```python
from build123d import *

# Parameters (mm, degrees)
SKETCH2_R                = 48.5
BOSS_EXTRUDE1_DEPTH      = 4
SKETCH4_R                = 1.5
CUT_EXTRUDE2_DEPTH       = 5
SKETCH5_R                = 3.75
CUT_EXTRUDE3_DEPTH       = 1.5
BOSS_EXTRUDE2_DEPTH      = 14
CUT_EXTRUDE5_REACH       = 44.5
SKETCH9_R                = 1.3
CUT_EXTRUDE6_DEPTH       = 7.5
CUT_EXTRUDE9_REACH       = 46.5
SKETCH11_R               = 9
BOSS_EXTRUDE7_DEPTH      = 9
BOSS_EXTRUDE7_DEPTH_BACK = 14
BOSS_EXTRUDE10_DEPTH     = 9
SKETCH27_W               = 16
SKETCH27_H               = 6
BOSS_EXTRUDE11_DEPTH     = 12
FILLET6_R                = 3
CUT_EXTRUDE16_REACH      = 75.05
SKETCH28_W               = 8
SKETCH28_H               = 4
CUT_EXTRUDE17_DEPTH      = 49.5
CUT_EXTRUDE17_DEPTH_BACK = 49.5
CROQUIS4_W               = 5.1
CROQUIS4_H               = 22.5
SALIENTE_EXTRUIR1_DEPTH  = 45
CROQUIS5_W               = 1.7
CROQUIS5_H               = 19.2
CORTAR_EXTRUIR1_DEPTH    = 19.5
CROQUIS6_W               = 18
CROQUIS6_H               = 17.447039648
CORTAR_EXTRUIR2_DEPTH    = 19.5
REDONDEO1_R              = 3
CROQUIS7_R               = 1.99
CORTAR_EXTRUIR3_DEPTH    = 10
CROQUIS8_W               = 0.564126112
CROQUIS8_H               = 2.164439882
SALIENTE_EXTRUIR2_DEPTH  = 3


with BuildPart() as part:
    # Sketch2 → Boss-Extrude1 (new body)
    with BuildSketch(Plane(origin=(0, 0, 0), x_dir=(1, 0, 0), z_dir=(0, 1, 0))):
        Circle(SKETCH2_R)
    extrude(amount=BOSS_EXTRUDE1_DEPTH)

    # Sketch4 → Cut-Extrude2 (cut, through all)
    with BuildSketch(Plane.XZ):
        with Locations((0, 7.25)):
            Circle(SKETCH4_R)
        with Locations((0, -7.25)):
            Circle(SKETCH4_R)
    extrude(amount=-CUT_EXTRUDE2_DEPTH, mode=Mode.SUBTRACT)

    # Sketch5 → Cut-Extrude3 (cut)
    with BuildSketch(Plane.XZ):
        Circle(SKETCH5_R)
    extrude(amount=-CUT_EXTRUDE3_DEPTH, mode=Mode.SUBTRACT)

    # Sketch7 → Boss-Extrude2 (add)
    with BuildSketch(Plane(origin=(-4, 0, 0), x_dir=(0, 0, -1), z_dir=(1, 0, 0))):
        with BuildLine():
            Line((23.129947874, 4), (23.129947874, 11.644549616))
            ThreePointArc((23.129947874, 11.644549616), (24.589048403, 18.743749901), (28.729797284, 24.692011643))
            ThreePointArc((28.729797284, 24.692011643), (29.313383054, 55.284736897), (-1.284289494, 55.479275971))
            Line((-1.284289494, 55.479275971), (-27.227315747, 29.536249718))
            ThreePointArc((-27.227315747, 29.536249718), (-32.64663453, 21.425665997), (-34.549646217, 11.858580188))
            Line((-34.549646217, 11.858580188), (-34.549646217, 4))
            Line((-34.549646217, 4), (23.129947874, 4))
        make_face()
    extrude(amount=-BOSS_EXTRUDE2_DEPTH)

    # Sketch8 → Cut-Extrude5 (cut, up to next)
    with BuildSketch(Plane(origin=(-6, 0, 0), x_dir=(0, 0, -1), z_dir=(1, 0, 0)), mode=Mode.PRIVATE) as cut_extrude5_sk1:
        Polygon((-15.249648422, 25.957567857), (13.741729607, 54.948945886), (28.590972012, 40.099703481), (-0.400406017, 11.108325452), align=None)
    cut_extrude5_tool1 = extrude(cut_extrude5_sk1.sketch, amount=-CUT_EXTRUDE5_REACH, mode=Mode.PRIVATE) & part.part
    add(cut_extrude5_tool1.solids().sort_by_distance((-6, 33.028636, -6.670662))[0], mode=Mode.SUBTRACT)

    # Sketch9 → Cut-Extrude6 (cut)
    with BuildSketch(Plane.ZY.offset(18)):
        with Locations((-20.105690637, 53.534732323)):
            Circle(SKETCH9_R)
        with Locations((-27.176758449, 46.463664511)):
            Circle(SKETCH9_R)
        with Locations((6.764367048, 12.522539014)):
            Circle(SKETCH9_R)
        with Locations((13.83543486, 19.593606826)):
            Circle(SKETCH9_R)
    extrude(amount=-CUT_EXTRUDE6_DEPTH, mode=Mode.SUBTRACT)

    # Sketch11 → Cut-Extrude9 (cut, up to next)
    with BuildSketch(Plane(origin=(-4, 0, 0), x_dir=(0, 0, -1), z_dir=(1, 0, 0)), mode=Mode.PRIVATE) as cut_extrude9_sk1:
        with Locations((13.918506302, 40.276480176)):
            Circle(SKETCH11_R)
    cut_extrude9_tool1 = extrude(cut_extrude9_sk1.sketch, amount=-CUT_EXTRUDE9_REACH, mode=Mode.PRIVATE) & part.part
    add(cut_extrude9_tool1.solids().sort_by_distance((-4, 40.27648, -13.918506))[0], mode=Mode.SUBTRACT)

    # Sketch17 → Boss-Extrude7 (add, two sides)
    with BuildSketch(Plane.ZY.offset(18)) as boss_extrude7_sk:
        with BuildLine():
            ThreePointArc((34.549646217, 11.858580188), (33.008342843, 20.500891953), (28.574482006, 28.077569775))
            ThreePointArc((28.574482006, 28.077569775), (27.915386359, 28.820289685), (27.227315747, 29.536249718))
            Line((27.227315747, 29.536249718), (1.284289494, 55.479275971))
            Line((1.284289494, 55.479275971), (26.295003593, 26.127182305))
            ThreePointArc((26.295003593, 26.127182305), (30.194232218, 19.461281607), (31.549646217, 11.858580188))
            Line((31.549646217, 11.858580188), (31.549646217, 4))
            Line((31.549646217, 4), (34.549646217, 4))
            Line((34.549646217, 4), (34.549646217, 11.858580188))
        make_face()
        with BuildLine():
            Line((28.574482006, 28.077569775), (3.405609837, 57.600596315))
            ThreePointArc((3.405609837, 57.600596315), (-31.461505391, 57.378912253), (-30.796489049, 22.517434639))
            ThreePointArc((-30.796489049, 22.517434639), (-27.345864981, 17.560549854), (-26.129947874, 11.644549616))
            Line((-26.129947874, 11.644549616), (-26.129947874, 4))
            Line((-26.129947874, 4), (-23.129947874, 4))
            Line((-23.129947874, 4), (-23.129947874, 11.644549616))
            ThreePointArc((-23.129947874, 11.644549616), (-24.589048403, 18.743749901), (-28.729797284, 24.692011643))
            ThreePointArc((-28.729797284, 24.692011643), (-29.313383054, 55.284736897), (1.284289494, 55.479275971))
            Line((1.284289494, 55.479275971), (27.227315747, 29.536249718))
            ThreePointArc((27.227315747, 29.536249718), (27.915386359, 28.820289685), (28.574482006, 28.077569775))
        make_face()
    extrude(amount=BOSS_EXTRUDE7_DEPTH)
    extrude(boss_extrude7_sk.sketch, amount=-BOSS_EXTRUDE7_DEPTH_BACK)

    # Sketch25 → Boss-Extrude10 (add)
    with BuildSketch(Plane.ZY.offset(18)):
        with BuildLine():
            ThreePointArc((-28.729797284, 24.692011643), (-24.589048403, 18.743749901), (-23.129947874, 11.644549616))
            Line((-23.129947874, 11.644549616), (-23.129947874, 4))
            Line((-23.129947874, 4), (-15.129947874, 4))
            add(Edge.make_bspline(
                [(-28.729797284, 24.692011643), (-21.954867515, 18.253200081), (-19.09405247, 12.798017691), (-15.129947874, 4)],
                knots=[0, 0, 0, 0, 1, 1, 1, 1], degree=3))
        make_face()
        with BuildLine():
            add(Edge.make_bspline(
                [(11.751619577, 43.19501844), (26.551255916, 25.8264495), (25.549646217, 4)],
                knots=[0, 0, 0, 1, 1, 1], degree=2))
            Line((25.549646217, 4), (31.549646217, 4))
            Line((31.549646217, 4), (31.549646217, 11.858580188))
            ThreePointArc((31.549646217, 11.858580188), (30.194232218, 19.461281607), (26.295003593, 26.127182305))
            Line((26.295003593, 26.127182305), (11.751619577, 43.19501844))
        make_face()
    extrude(amount=BOSS_EXTRUDE10_DEPTH)

    # Sketch27 → Boss-Extrude11 (add)
    with BuildSketch(Plane(origin=(0, 4, 0), x_dir=(1, 0, 0), z_dir=(0, 1, 0))):
        with Locations((6, -21.549646217)):
            Rectangle(SKETCH27_W, SKETCH27_H)
    extrude(amount=BOSS_EXTRUDE11_DEPTH)

    # Fillet6
    fillet6_edges = [part.edges().sort_by_distance(p)[0] for p in [
        (-2, 16, 21.549646217),
        (14, 16, 21.549646217),
    ]]
    fillet(fillet6_edges, radius=FILLET6_R)

    # Sketch28 → Cut-Extrude16 (cut, up to next)
    with BuildSketch(Plane.XY.offset(24.549646217), mode=Mode.PRIVATE) as cut_extrude16_sk1:
        with Locations((6, 10)):
            Rectangle(SKETCH28_W, SKETCH28_H)
    cut_extrude16_tool1 = extrude(cut_extrude16_sk1.sketch, amount=-CUT_EXTRUDE16_REACH, mode=Mode.PRIVATE) & part.part
    add(cut_extrude16_tool1.solids().sort_by_distance((6, 10, 24.549646))[0], mode=Mode.SUBTRACT)

    # Sketch29 → Cut-Extrude17 (cut, two sides)
    with BuildSketch(Plane.XY) as cut_extrude17_sk:
        with BuildLine():
            Line((-21, 64.776480176), (-27, 64.776480176))
            Line((-27, 64.776480176), (-27, 4))
            Line((-27, 4), (-26.5, 4))
            add(Edge.make_bspline(
                [(-21, 64.776480176), (-21.220459696, 34.140901434), (-26.5, 4)],
                knots=[0, 0, 0, 1, 1, 1], degree=2))
        make_face()
    extrude(amount=CUT_EXTRUDE17_DEPTH, mode=Mode.SUBTRACT)
    extrude(cut_extrude17_sk.sketch, amount=-CUT_EXTRUDE17_DEPTH_BACK, mode=Mode.SUBTRACT)

    # Croquis4 → Saliente-Extruir1 (add)
    with BuildSketch(Plane(origin=(0, 4, 0), x_dir=(1, 0, 0), z_dir=(0, 1, 0))):
        with Locations((35, 13.919947874)):
            Rectangle(CROQUIS4_W, CROQUIS4_H)
    extrude(amount=SALIENTE_EXTRUIR1_DEPTH)

    # Croquis5 → Cortar-Extruir1 (cut)
    with BuildSketch(Plane(origin=(0, 49, 0), x_dir=(1, 0, 0), z_dir=(0, 1, 0))):
        with Locations((35, 13.919947874)):
            Rectangle(CROQUIS5_W, CROQUIS5_H)
    extrude(amount=-CORTAR_EXTRUIR1_DEPTH, mode=Mode.SUBTRACT)

    # Croquis6 → Cortar-Extruir2 (cut)
    with BuildSketch(Plane(origin=(37.55, 0, 0), x_dir=(0, 0, -1), z_dir=(1, 0, 0))):
        with Locations((13.918506302, 40.276480176)):
            Rectangle(CROQUIS6_W, CROQUIS6_H)
    extrude(amount=-CORTAR_EXTRUIR2_DEPTH, mode=Mode.SUBTRACT)

    # Redondeo1
    redondeo1_edges = [part.edges().sort_by_distance(p)[0] for p in [
        (32.45, 4, -13.919947874),
        (35, 4, -2.669947874),
    ]]
    fillet(redondeo1_edges, radius=REDONDEO1_R)

    # Croquis7 → Cortar-Extruir3 (cut)
    with BuildSketch(Plane.XZ.offset(-1.5)):
        Circle(CROQUIS7_R)
    extrude(amount=-CORTAR_EXTRUIR3_DEPTH, mode=Mode.SUBTRACT)

    # Croquis8 → Saliente-Extruir2 (add)
    with BuildSketch(Plane.XZ.offset(-1.5)):
        with Locations((-1.952063056, 0)):
            Rectangle(CROQUIS8_W, CROQUIS8_H)
    extrude(amount=-SALIENTE_EXTRUIR2_DEPTH)


solid = part.part
```
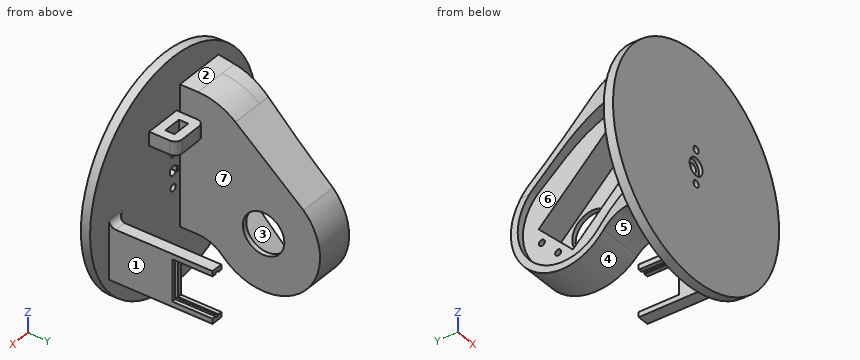
Source: CAD feature listing. Evaluate the final solid. Frame: model axes, mm. Face numbers are marked on the shaded views. A direction names the side the tool comes from. Round coordinates to 2 decimals unless told otherwise and drop trailing zeros. Write each loop counter-clockwise with the first axis right and the second up, starting at its lowest first coordinate (ties: lowest second). Pieces come first, ordered by that corner, then holes. Notation, with made-up numbers: M 56,47 L 88,47 A17 cw 88,61 Z; hole C 35,43 d7. An arc over 180 degrees is marked long. Use CSV: the item, a comma, the result in double quotes. Start each with the question number.
Q1. First-contact query: P1, Ø13, axis at x = 6, y = 7.5, coming from the +Z side; P2, Ø8, axis at x = -22.5, z = 33.5, coming from the +Y side; P3, Ø8, axis at y = 24.5, z = -8.5, coming from the +X side. Flat tips, straight axial feed; report the tip coordinate or a pass-through.
Q2. Cut plane B-B on z = -7.25. Count the separate pieces of the cut face and the enclosed holes in it, plus the area to 3 significant figures.
Q3. Pull-direction query (X, two-part tool) for the marked faces 5, 6 and 7; classes: +X half, -X half, draft (parallel to the pull), parting line (faces both ways), or undercut.
Q4. Cut plane A-A on x = 26.5. Output: boundary loops of the cut face in (y, z), plus the area to 3 significant figures.
Q5. Access query for the marked faces 1, 2, 3 and 4. Directions: +Z, -Z, +X, -X, +Y, -Y. A direction counts if a zero-diameter tool reaches every point of the face in a straight line with its end or side. Return the directions, or none.
Q6. Line query: line 1 (Z direction, x = 0, y = 2.6); line 2 (Z direction, x = 0, y = 0.9); line 3 (Y direction, x = 19.5, z = 11). Output: solid intervals per line, ascending. Write a range as from..to.
Results found:
1,P1,"z = 48.5"
1,P2,"y = 26.92"
1,P3,"x = 37.55"
2,separate pieces,"3"
2,enclosed holes,"0"
2,area,"977 mm^2"
3,face 5,"draft"
3,face 6,"-X half"
3,face 7,"undercut"
4,outline,"M 0,-40.62 L 4,-40.62 L 4,40.62 L 0,40.62 Z"
4,area,"325 mm^2"
5,face 1,"+Z, -Z, +X, +Y"
5,face 2,"+Z, +X, -X, +Y"
5,face 3,"-X"
5,face 4,"+X, -X"
6,line 1,"-48.5..-8.75, -5.75..-1.99, 1.99..5.75, 8.75..48.5"
6,line 2,"-48.5..-8.75, -5.75..-3.75, 3.75..5.75, 8.75..48.5"
6,line 3,"0..4"
